```python
from build123d import *

# Parameters (mm, degrees)
SKETCH1_W           = 100
SKETCH1_H           = 100
BOSS_EXTRUDE1_DEPTH = 2.5
SKETCH5_W           = 87
SKETCH5_H           = 87
CUT_EXTRUDE2_DEPTH  = 4
SKETCH6_R           = 15
BOSS_EXTRUDE3_DEPTH = 2.5
SKETCH7_W           = 15.5
SKETCH7_H           = 15.5
CUT_EXTRUDE3_DEPTH  = 2.5
BOSS_EXTRUDE4_DEPTH = 2.5
EXTRUDE_THIN2_DEPTH = 2.5
SKETCH10_R          = 3
CUT_EXTRUDE5_DEPTH  = 2.5
SKETCH11_R          = 6.5
BOSS_EXTRUDE5_DEPTH = 2.5
SKETCH12_R          = 3
CUT_EXTRUDE6_DEPTH  = 3
SKETCH13_R          = 7
SKETCH13_R_2        = 5
BOSS_EXTRUDE6_DEPTH = 2.5
SKETCH14_W          = 5
SKETCH14_H          = 9
EXTRUDE_THIN5_DEPTH = 2.5
SKETCH15_W          = 17.095160315
SKETCH15_H          = 3.5
EXTRUDE_THIN7_DEPTH = 2.5
BOSS_EXTRUDE8_DEPTH = 2.5
SKETCH20_W          = 31.082582927
SKETCH20_H          = 6.049047595
CUT_EXTRUDE8_DEPTH  = 2.5
SKETCH21_R          = 3
CUT_EXTRUDE9_DEPTH  = 10


with BuildPart() as part:
    # Sketch1 → Boss-Extrude1 (new body)
    with BuildSketch(Plane(origin=(0, 0, 0), x_dir=(1, 0, 0), z_dir=(0, 1, 0))):
        Rectangle(SKETCH1_W, SKETCH1_H)
    extrude(amount=BOSS_EXTRUDE1_DEPTH)

    # Sketch5 → Cut-Extrude2 (cut)
    with BuildSketch(Plane(origin=(0, 2.5, 0), x_dir=(1, 0, 0), z_dir=(0, 1, 0))):
        Rectangle(SKETCH5_W, SKETCH5_H)
    extrude(amount=-CUT_EXTRUDE2_DEPTH, mode=Mode.SUBTRACT)

    # Sketch8 → Boss-Extrude4 (add)
    with BuildSketch(Plane(origin=(0, 2.5, 0), x_dir=(1, 0, 0), z_dir=(0, 1, 0))):
        with BuildLine():
            Line((-43.5, -43.5), (-30.220069463, -43.5))
            ThreePointArc((-30.220069463, -43.5), (-34.109671064, -34.109671064), (-43.5, -30.220069463))
            Line((-43.5, -30.220069463), (-43.5, -43.5))
        make_face()
        with BuildLine():
            ThreePointArc((-43.5, 30.220069463), (-34.109671064, 34.109671064), (-30.220069463, 43.5))
            Line((-30.220069463, 43.5), (-43.5, 43.5))
            Line((-43.5, 43.5), (-43.5, 30.220069463))
        make_face()
        with BuildLine():
            Line((43.5, 43.5), (30.220069463, 43.5))
            ThreePointArc((30.220069463, 43.5), (34.109671064, 34.109671064), (43.5, 30.220069463))
            Line((43.5, 30.220069463), (43.5, 43.5))
        make_face()
        with BuildLine():
            ThreePointArc((43.5, -30.220069463), (34.109671064, -34.109671064), (30.220069463, -43.5))
            Line((30.220069463, -43.5), (43.5, -43.5))
            Line((43.5, -43.5), (43.5, -30.220069463))
        make_face()
    extrude(amount=-BOSS_EXTRUDE4_DEPTH)



with BuildPart() as body_2:
    # Sketch6 → Boss-Extrude3 (new body)
    with BuildSketch(Plane(origin=(0, 2.5, 0), x_dir=(1, 0, 0), z_dir=(0, 1, 0))):
        with Locations(Location((0, 0, 0), (0, 0, 270))):
            Circle(SKETCH6_R)
    extrude(amount=-BOSS_EXTRUDE3_DEPTH)

    # Sketch7 → Cut-Extrude3 (cut)
    with BuildSketch(Plane(origin=(0, 2.5, 0), x_dir=(1, 0, 0), z_dir=(0, 1, 0))):
        Rectangle(SKETCH7_W, SKETCH7_H)
    extrude(amount=-CUT_EXTRUDE3_DEPTH, mode=Mode.SUBTRACT)


with BuildPart() as part_1:
    add(part.part)

    add(body_2.part)  # Extrude-Thin2 merges body 2
    # Sketch9 → Extrude-Thin2 (add)
    with BuildSketch(Plane(origin=(0, 2.5, 0), x_dir=(1, 0, 0), z_dir=(0, 1, 0))):
        Polygon((4.214466094, -11.285533906), (34.46870341, -41.539771222), (41.539771222, -34.46870341), (11.285533906, -4.214466094), align=None)
        Polygon((-11.285533906, -4.214466094), (-41.539771222, -34.46870341), (-34.46870341, -41.539771222), (-4.214466094, -11.285533906), align=None)
        Polygon((11.285533906, 4.214466094), (41.539771222, 34.46870341), (34.46870341, 41.539771222), (4.214466094, 11.285533906), align=None)
        Polygon((-4.214466094, 11.285533906), (-34.46870341, 41.539771222), (-41.539771222, 34.46870341), (-11.285533906, 4.214466094), align=None)
    extrude(amount=-EXTRUDE_THIN2_DEPTH)

    # Sketch10 → Cut-Extrude5 (cut)
    with BuildSketch(Plane(origin=(0, 2.5, 0), x_dir=(1, 0, 0), z_dir=(0, 1, 0))):
        with Locations(Location((36, 36, 0), (0, 0, 270))):
            Circle(SKETCH10_R)
        with Locations(Location((-36, 36, 0), (0, 0, 90))):
            Circle(SKETCH10_R)
        with Locations(Location((36, -36, 0), (0, 0, 90))):
            Circle(SKETCH10_R)
        with Locations(Location((-36, -36, 0), (0, 0, 270))):
            Circle(SKETCH10_R)
    extrude(amount=-CUT_EXTRUDE5_DEPTH, mode=Mode.SUBTRACT)

    # Sketch11 → Boss-Extrude5 (add)
    with BuildSketch(Plane(origin=(0, 2.5, 0), x_dir=(1, 0, 0), z_dir=(0, 1, 0))):
        with Locations((0, -43.5)):
            Circle(SKETCH11_R)
        with Locations((0, 43.5)):
            Circle(SKETCH11_R)
    extrude(amount=-BOSS_EXTRUDE5_DEPTH)

    # Sketch12 → Cut-Extrude6 (cut)
    with BuildSketch(Plane(origin=(0, 2.5, 0), x_dir=(1, 0, 0), z_dir=(0, 1, 0))):
        with Locations(Location((0, 43.5, 0), (0, 0, 270))):
            Circle(SKETCH12_R)
        with Locations(Location((0, -43.5, 0), (0, 0, 270))):
            Circle(SKETCH12_R)
    extrude(amount=-CUT_EXTRUDE6_DEPTH, mode=Mode.SUBTRACT)



with BuildPart() as body_2_2:
    # Sketch13 → Boss-Extrude6 (new body)
    with BuildSketch(Plane(origin=(0, 2.5, 0), x_dir=(1, 0, 0), z_dir=(0, 1, 0))):
        with Locations(Location((0, 26.5, 0), (0, 0, 270))):
            Circle(SKETCH13_R)
        with Locations(Location((0, 26.5, 0), (0, 0, 270))):
            Circle(SKETCH13_R_2, mode=Mode.SUBTRACT)
    extrude(amount=-BOSS_EXTRUDE6_DEPTH)


with BuildPart() as part_2:
    add(part_1.part)

    add(body_2_2.part)  # Extrude-Thin5 merges body 2 2
    # Sketch14 → Extrude-Thin5 (add)
    with BuildSketch(Plane(origin=(0, 0, 0), x_dir=(-1, 0, 0), z_dir=(0, -1, 0))):
        with Locations((0, 36)):
            Rectangle(SKETCH14_W, SKETCH14_H)
    extrude(amount=-EXTRUDE_THIN5_DEPTH)

    # Sketch15 → Extrude-Thin7 (add)
    with BuildSketch(Plane(origin=(0, 0, 0), x_dir=(-1, 0, 0), z_dir=(0, -1, 0))):
        with Locations((-13.979094467, 26.5)):
            Rectangle(SKETCH15_W, SKETCH15_H)
        with Locations((13.979094467, 26.5)):
            Rectangle(SKETCH15_W, SKETCH15_H)
    extrude(amount=-EXTRUDE_THIN7_DEPTH)

    # Sketch17 → Boss-Extrude8 (add)
    with BuildSketch(Plane(origin=(0, 0, 0), x_dir=(-1, 0, 0), z_dir=(0, -1, 0))):
        with BuildLine():
            Line((6.591379734, 37.425929606), (-6.591379734, 37.425929606))
            ThreePointArc((-6.591379734, 37.425929606), (-15.665450128, 46.5), (-6.591379734, 55.574070394))
            Line((-6.591379734, 55.574070394), (6.591379734, 55.574070394))
            ThreePointArc((6.591379734, 55.574070394), (15.665450128, 46.5), (6.591379734, 37.425929606))
        make_face()
    extrude(amount=-BOSS_EXTRUDE8_DEPTH)

    # Sketch20 → Cut-Extrude8 (cut)
    with BuildSketch(Plane(origin=(0, 0, 0), x_dir=(-1, 0, 0), z_dir=(0, -1, 0))):
        with Locations((-0.578009107, 53.024523798)):
            Rectangle(SKETCH20_W, SKETCH20_H)
    extrude(amount=-CUT_EXTRUDE8_DEPTH, mode=Mode.SUBTRACT)

    # Sketch21 → Cut-Extrude9 (cut)
    with BuildSketch(Plane(origin=(0, 0, 0), x_dir=(-1, 0, 0), z_dir=(0, -1, 0))):
        with Locations(Location((0, 40.5, 0), (0, 0, 90))):
            Circle(SKETCH21_R)
    extrude(amount=-CUT_EXTRUDE9_DEPTH, mode=Mode.SUBTRACT)


solid = part_2.part
```
The model under review builds one solid part; all positions refer to its coordinate system, in mm. Coordinates: 2 decimals unless noted, no trailing zeros. Write each loop counter-clockwise with the first axis right and the second up, starting at its lowest first coordinate (ties: lowest second). Pieces come first, ordered by that corner, then holes.
1) Clearance check with a flat-ended pin moving along its axis: pin 1 Ø12 at (x, z) = (-34, -13) entering from -Y. State where the tip first meets the part, or that it passes through.
2) We need section D-D on z = -36. State the section outline as (x, y) points.
3) We need section C-C on x = 0. State the section outline as (y, z) points, then the cut area to 3 significant figures.
4) We need section A-A on x = -26.5. State the section outline as (y, z) points.
5) The part is to be moulded in two halves that separate along X. For faces 1 (the face through (-1, 2.5, -12)), 2 (the face through (12.15, 1.27, -19.22)), say which applies: pulls with the +X half, pulls with the -X half, needs draft (parallel to the pull), parting line crosses it, or undercut.
6) To check wall thickness, follow probe 1 along X at (y, z) = (2.2, 42); probe 2 along X at (y, z) = (1.8, -20.5); probe 3 along X at (y, z) = (1.7, 10). State the ranges of each line that lie inside material, in increasing order.
7) We need section B-B on z = 28. State the section outline as (x, y) points.
Answer list:
1. pin 1: passes through
2. outline: (-50, 0) - (-39, 0) - (-39, 2.5) - (-50, 2.5) - close; (-33, 0) - (-28.93, 0) - (-28.93, 2.5) - (-33, 2.5) - close; (-2.5, 0) - (2.5, 0) - (2.5, 2.5) - (-2.5, 2.5) - close; (28.93, 0) - (33, 0) - (33, 2.5) - (28.93, 2.5) - close; (39, 0) - (50, 0) - (50, 2.5) - (39, 2.5) - close
3. outline: (0, -50) - (2.5, -50) - (2.5, -43.5) - (0, -43.5) - close; (0, -37.5) - (2.5, -37.5) - (2.5, -31.5) - (0, -31.5) - close; (0, -21.5) - (2.5, -21.5) - (2.5, -19.5) - (0, -19.5) - close; (0, -15) - (2.5, -15) - (2.5, -7.75) - (0, -7.75) - close; (0, 7.75) - (2.5, 7.75) - (2.5, 15) - (0, 15) - close; (0, 37) - (2.5, 37) - (2.5, 40.5) - (0, 40.5) - close; (0, 46.5) - (2.5, 46.5) - (2.5, 50) - (0, 50) - close
3. area: 90.0 mm2
4. outline: (0, -50) - (2.5, -50) - (2.5, -43.5) - (0, -43.5) - close; (0, -33.57) - (2.5, -33.57) - (2.5, -19.43) - (0, -19.43) - close; (0, 19.43) - (2.5, 19.43) - (2.5, 33.57) - (0, 33.57) - close; (0, 43.5) - (2.5, 43.5) - (2.5, 50) - (0, 50) - close
5. face 1: needs draft
5. face 2: undercut
6. probe 1: x = -50 to -30.31, -6.32 to -2.6, 2.6 to 6.32, 30.31 to 50
6. probe 2: x = -50 to -43.5, -27.57 to -13.43, -3.61 to 3.61, 13.43 to 27.57, 43.5 to 50
6. probe 3: x = -50 to -43.5, -17.07 to 17.07, 43.5 to 50
7. outline: (-50, 0) - (-43.5, 0) - (-43.5, 2.5) - (-50, 2.5) - close; (-35.07, 0) - (-20.93, 0) - (-20.93, 2.5) - (-35.07, 2.5) - close; (20.93, 0) - (35.07, 0) - (35.07, 2.5) - (20.93, 2.5) - close; (43.5, 0) - (50, 0) - (50, 2.5) - (43.5, 2.5) - close
